Geometry: see drawing. Coordinates: mm, zero at the bounding-box minimum. A direction names the side the tool comes from. Round coordinates to 2 decimals unless told otherwise and drop trailing zeros. Write each loop counter-clockwise with the first axis right and the second up, starting at its lowest first coordinate (ties: lowest second). Pieces come first, ordered by that corner, then holes. Notation, with made-up numbers: (59.25, 82) -> (74.25, 82) arc R3 cw to (74.25, 86) -> close; hole circle Ø11 at (1, 43.25). An arc over 180 degrees is marked (long way). Use CSV: the item, a comma, the result in double quotes.
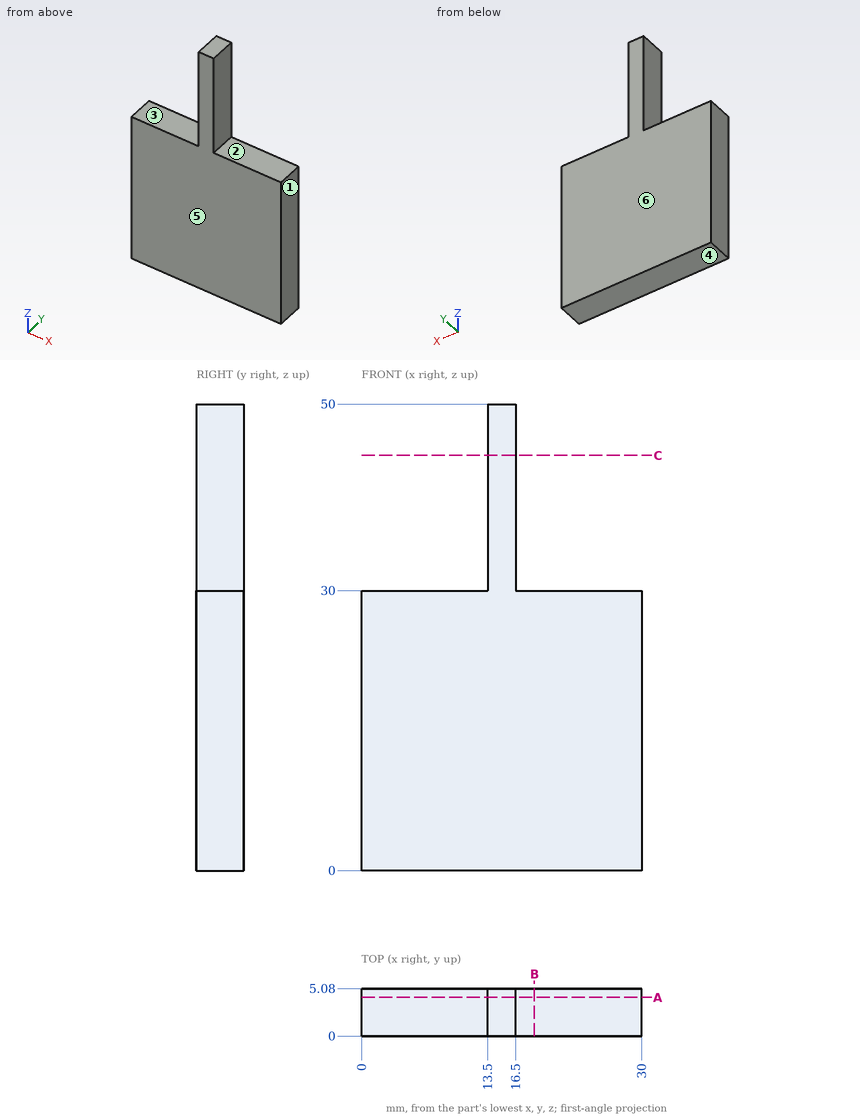
Item 1: Section query A-A on y = 4.15. Return the cut outline in (x, z).
Worked answers:
outline,"(0, 0) -> (30, 0) -> (30, 30) -> (16.5, 30) -> (16.5, 50) -> (13.5, 50) -> (13.5, 30) -> (0, 30) -> close"
Item 2: Line query: line 1 (Z direction, x = 11.5, y = 1.25); line 2 (X direction, y = 1.85, z = 42.5). Output: solid intervals per line, ascending.
Worked answers:
line 1,"z = 0 to 30"
line 2,"x = 13.5 to 16.5"
Item 3: Set-up query: the marked faces 1, 2 and 3. Return all of +Z, -Z, +X, -X, +Y, -Y with unobstructed straight access to the full face (end or side cutting, diameter ignored); none if empty.
Worked answers:
face 1,"+Z, -Z, +X, +Y, -Y"
face 2,"+Z, +X, +Y, -Y"
face 3,"+Z, -X, +Y, -Y"
Item 4: Section query B-B on x = 18.5. Return the cut outline in (y, z).
Worked answers:
outline,"(0, 0) -> (5.08, 0) -> (5.08, 30) -> (0, 30) -> close"
Item 5: First-contact query: pin 1 Ø2.5 at (y, z) = (2.5, 40.5) entering from -X; pin 2 Ø1.5 at (x, y) = (24.5, 1.5) entering from +Z. Flat tips, straight axial feed; report the tip coordinate or a pass-through.
Worked answers:
pin 1,"stops at x = 13.5"
pin 2,"stops at z = 30"
Item 6: Section query C-C on z = 44.5. Return the cut outline in (x, y).
Worked answers:
outline,"(13.5, 0) -> (16.5, 0) -> (16.5, 5.08) -> (13.5, 5.08) -> close"
Item 7: Pull-direction query (Y, two-part tool) for the marked faces 4, 5 and 6; classes: +Y half, -Y half, draft (parallel to the pull), parting line (faces both ways), or undercut.
Worked answers:
face 4,"draft"
face 5,"-Y half"
face 6,"+Y half"
